Source: CAD feature listing. Evaluate the final solid. Frame: model axes, mm. Face numbers are marked on the shaded views. A direction names the side the tool comes from. Round coordinates to 2 decimals unless told otherwise and drop trailing zeros. Write each loop counter-clockwise with the first axis right and the second up, starting at its lowest first coordinate (ties: lowest second). Pieces come first, ordered by that corner, then holes. Notation, with made-up numbers: M 62.25,83.25 L 86.25,83.25 A15 cw 86.25,97.25 Z; hole C 79,-24.75 d5. An arc over 180 degrees is marked long. Answer in a Markdown table with one row per item. Add a question column.
Item 1: Mould query, pull axis Y, two halves, no side actions, for the marked faces 3 and 4. Classes: released by +Y, released by -Y, zero draft, split by the parting line, or undercut.
Item 2: Contact query for flat-ended pins moving along their axis: pin 1 (1 mm diameter, centred on x = 1, z = -6.5, fed in from -Y); pin 2 (3 mm diameter, centred on x = 2, y = 7, fed in from +Z); pin 3 (3 mm diameter, centred on x = 1.5, z = 8.5, fed in from +Y). Output: stop coordinate, or through.
Item 3: Cut plane C-C on x = 1.7. Return loops of the section in (y, z).
Item 4: Material intervals for probe 1 along Z at (x, y) = (3.8, 0); probe 2 along Z at (x, y) = (4.9, 0); probe 3 along X at (y, z) = (-7.75, 7), sorted ascending.
Item 5: Set-up query: the marked faces 1 and 2. Return all of +Z, -Z, +X, -X, +Y, -Y with unobstructed straight access to the full face (end or side cutting, diameter ignored); none if empty.
from build123d import *

# Parameters (mm, degrees)
FILLET1_R = 0.3


with BuildPart() as part:
    # Sketch1 → Revolve1 (revolve)
    with BuildSketch(Plane.XY, mode=Mode.PRIVATE) as revolve1_sk:
        Polygon((0, 7.5), (0, 8.5), (0.25, 8.5), (0.25, 11.1), (0, 11.1), (0, 12), (5, 12), (5, 11.1), (4.75, 11.1), (4.75, 8.5), (5, 8.5), (5, 7.5), align=None)
    revolve(revolve1_sk.sketch.rotate(Axis((0, 0, 0), (1, 0, 0)), 180), axis=Axis((0, 0, 0), (1, 0, 0)))

    # Fillet1
    fillet1_edges = [part.edges().sort_by_distance(p)[0] for p in [
        (5, 12, 0),
        (0, 12, 0),
        (0, 7.5, 0),
        (5, 7.5, 0),
    ]]
    fillet(fillet1_edges, radius=FILLET1_R)


solid = part.part
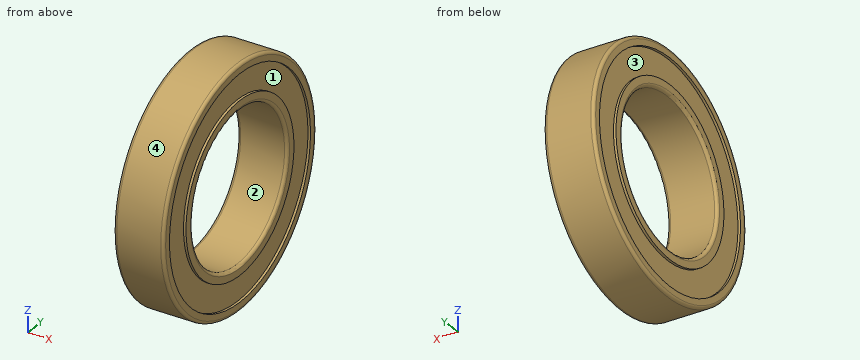
Results below:
| question | item | result |
|---|---|---|
| 1 | face 3 | undercut |
| 1 | face 4 | split by the parting line |
| 2 | pin 1 | y = -10.39 |
| 2 | pin 2 | z = 10.67 |
| 2 | pin 3 | y = 9.75 |
| 3 | outline | C 0,0 d24; hole C 0,0 d15 |
| 4 | probe 1 | -12 to -7.5, 7.5 to 12 |
| 4 | probe 2 | -11.92 to -11.1, -8.5 to -7.58, 7.58 to 8.5, 11.1 to 11.92 |
| 4 | probe 3 | 0.25 to 4.75 |
| 5 | face 1 | +X |
| 5 | face 2 | +X, -X |
